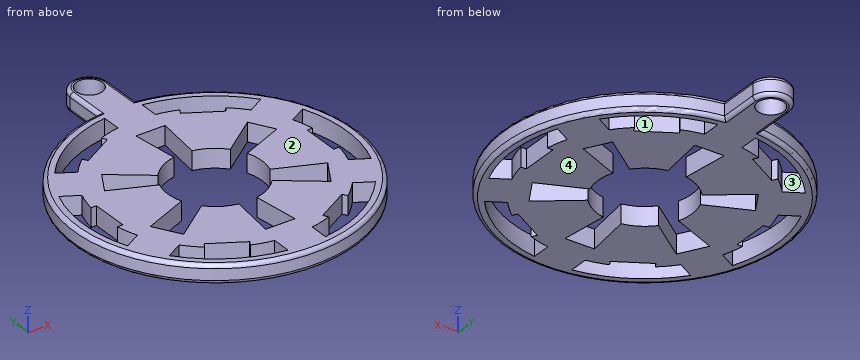
```python
from build123d import *

# Parameters (mm, degrees)
F1_DEPTH = 5
F0_R     = 3.5
F2_DEPTH = 5
F3_R     = 1


with BuildPart() as f1:
    # F0 (on Top) → F1 (new body)
    with BuildSketch(Plane.XY):
        with BuildLine():
            ThreePointArc((-4.988375268, 37.1667339456), (-24.6899364868, -28.2251135742), (37.5, 0))
            ThreePointArc((37.5, 0), (28.2251135742, 24.6899364868), (4.988375268, 37.1667339456))
            ThreePointArc((4.988375268, 37.1667339456), (0, 37.5), (-4.988375268, 37.1667339456))
        make_face()
        with BuildLine():
            Line((-5, -29.5803989155), (-5, -30))
            Line((-5, -30), (-5, -34.6410161514))
            ThreePointArc((-5, -34.6410161514), (-17.5, -30.3108891325), (-27.5, -21.6506350946))
            Line((-27.5, -21.6506350946), (-23.1173769149, -19.1203264767))
            ThreePointArc((-23.1173769149, -19.1203264767), (-21.2132034356, -21.2132034356), (-19.1203264767, -23.1173769149))
            Line((-19.1203264767, -23.1173769149), (-18.3888154764, -21.8503626961))
            Line((-18.3888154764, -21.8503626961), (-9.7285614385, -26.8503626961))
            Line((-9.7285614385, -26.8503626961), (-10.4600724388, -28.1173769149))
            ThreePointArc((-10.4600724388, -28.1173769149), (-7.7645713531, -28.9777747887), (-5, -29.5803989155))
        make_face(mode=Mode.SUBTRACT)
        with BuildLine():
            ThreePointArc((-32.5, -12.9903810568), (-35, 0), (-32.5, 12.9903810568))
            Line((-32.5, 12.9903810568), (-28.1173769149, 10.4600724388))
            ThreePointArc((-28.1173769149, 10.4600724388), (-28.9777747887, 7.7645713531), (-29.5803989155, 5))
            Line((-29.5803989155, 5), (-28.1173769149, 5))
            Line((-28.1173769149, 5), (-28.1173769149, -5))
            Line((-28.1173769149, -5), (-29.5803989155, -5))
            ThreePointArc((-29.5803989155, -5), (-28.9777747887, -7.7645713531), (-28.1173769149, -10.4600724388))
            Line((-28.1173769149, -10.4600724388), (-32.5, -12.9903810568))
        make_face(mode=Mode.SUBTRACT)
        with BuildLine():
            Line((5, -30), (5, -29.5803989155))
            ThreePointArc((5, -29.5803989155), (7.7645713531, -28.9777747887), (10.4600724388, -28.1173769149))
            Line((10.4600724388, -28.1173769149), (9.7285614385, -26.8503626961))
            Line((9.7285614385, -26.8503626961), (18.3888154764, -21.8503626961))
            Line((18.3888154764, -21.8503626961), (19.1203264767, -23.1173769149))
            ThreePointArc((19.1203264767, -23.1173769149), (21.2132034356, -21.2132034356), (23.1173769149, -19.1203264767))
            Line((23.1173769149, -19.1203264767), (27.5, -21.6506350946))
            ThreePointArc((27.5, -21.6506350946), (17.5, -30.3108891325), (5, -34.6410161514))
            Line((5, -34.6410161514), (5, -30))
        make_face(mode=Mode.SUBTRACT)
        with BuildLine():
            ThreePointArc((-9.6656079434, 7.926286841), (-6.3749366407, 10.7522175772), (-2.3166453596, 12.2834504223))
            Line((-2.3166453596, 12.2834504223), (-3.8166453596, 24.5))
            Line((-3.8166453596, 24.5), (4, 24.5))
            Line((4, 24.5), (2.5, 12.2474487139))
            ThreePointArc((2.5, 12.2474487139), (6.4551230926, 10.7042695154), (9.6656079434, 7.926286841))
            Line((9.6656079434, 7.926286841), (19.4529138373, 15.3065648785))
            Line((19.4529138373, 15.3065648785), (22.9823309481, 9.1934351215))
            Line((22.9823309481, 9.1934351215), (11.6971697336, 4.4075186015))
            ThreePointArc((11.6971697336, 4.4075186015), (12.4985113757, 0.1929077306), (11.827620909, -4.0444262427))
            Line((11.827620909, -4.0444262427), (23.6581671568, -9.040247023))
            Line((23.6581671568, -9.040247023), (19.6581671568, -15.9684502533))
            Line((19.6581671568, -15.9684502533), (9.4163863244, -8.2208070522))
            ThreePointArc((9.4163863244, -8.2208070522), (6.2891594451, -10.8026141963), (2.5, -12.2474487139))
            Line((2.5, -12.2474487139), (4, -24.5))
            Line((4, -24.5), (-3.8166453596, -24.5))
            Line((-3.8166453596, -24.5), (-2.3166453596, -12.2834504223))
            ThreePointArc((-2.3166453596, -12.2834504223), (-6.2082425785, -10.849319061), (-9.4163863244, -8.2208070522))
            Line((-9.4163863244, -8.2208070522), (-19.6581671568, -15.9684502533))
            Line((-19.6581671568, -15.9684502533), (-23.6581671568, -9.040247023))
            Line((-23.6581671568, -9.040247023), (-11.827620909, -4.0444262427))
            ThreePointArc((-11.827620909, -4.0444262427), (-12.4985113757, 0.1929077306), (-11.6971697336, 4.4075186015))
            Line((-11.6971697336, 4.4075186015), (-22.9823309481, 9.1934351215))
            Line((-22.9823309481, 9.1934351215), (-19.4529138373, 15.3065648785))
            Line((-19.4529138373, 15.3065648785), (-9.6656079434, 7.926286841))
        make_face(mode=Mode.SUBTRACT)
        with BuildLine():
            Line((28.1173769149, 10.4600724388), (32.5, 12.9903810568))
            ThreePointArc((32.5, 12.9903810568), (35, 0), (32.5, -12.9903810568))
            Line((32.5, -12.9903810568), (28.1173769149, -10.4600724388))
            ThreePointArc((28.1173769149, -10.4600724388), (28.9777747887, -7.7645713531), (29.5803989155, -5))
            Line((29.5803989155, -5), (28.1173769149, -5))
            Line((28.1173769149, -5), (28.1173769149, 5))
            Line((28.1173769149, 5), (29.5803989155, 5))
            ThreePointArc((29.5803989155, 5), (28.9777747887, 7.7645713531), (28.1173769149, 10.4600724388))
        make_face(mode=Mode.SUBTRACT)
        with BuildLine():
            Line((-5, 30), (-5, 29.5803989155))
            ThreePointArc((-5, 29.5803989155), (-7.7645713531, 28.9777747887), (-10.4600724388, 28.1173769149))
            Line((-10.4600724388, 28.1173769149), (-9.7285614385, 26.8503626961))
            Line((-9.7285614385, 26.8503626961), (-18.3888154764, 21.8503626961))
            Line((-18.3888154764, 21.8503626961), (-19.1203264767, 23.1173769149))
            ThreePointArc((-19.1203264767, 23.1173769149), (-21.2132034356, 21.2132034356), (-23.1173769149, 19.1203264767))
            Line((-23.1173769149, 19.1203264767), (-27.5, 21.6506350946))
            ThreePointArc((-27.5, 21.6506350946), (-17.5, 30.3108891325), (-5, 34.6410161514))
            Line((-5, 34.6410161514), (-5, 30))
        make_face(mode=Mode.SUBTRACT)
        with BuildLine():
            Line((5, 29.5803989155), (5, 30))
            Line((5, 30), (5, 34.6410161514))
            ThreePointArc((5, 34.6410161514), (17.5, 30.3108891325), (27.5, 21.6506350946))
            Line((27.5, 21.6506350946), (23.1173769149, 19.1203264767))
            ThreePointArc((23.1173769149, 19.1203264767), (21.2132034356, 21.2132034356), (19.1203264767, 23.1173769149))
            Line((19.1203264767, 23.1173769149), (18.3888154764, 21.8503626961))
            Line((18.3888154764, 21.8503626961), (9.7285614385, 26.8503626961))
            Line((9.7285614385, 26.8503626961), (10.4600724388, 28.1173769149))
            ThreePointArc((10.4600724388, 28.1173769149), (7.7645713531, 28.9777747887), (5, 29.5803989155))
        make_face(mode=Mode.SUBTRACT)
    extrude(amount=F1_DEPTH)

    # F0 (on Top) → F2 (join)
    with BuildSketch(Plane.XY):
        with BuildLine():
            ThreePointArc((-4.988375268, 37.1667339456), (0, 37.5), (4.988375268, 37.1667339456))
            Line((4.988375268, 37.1667339456), (4.988375268, 47.2334879431))
            ThreePointArc((4.988375268, 47.2334879431), (0, 42.5045103852), (-4.988375268, 47.2334879431))
            Line((-4.988375268, 47.2334879431), (-4.988375268, 37.1667339456))
        make_face()
        with BuildLine():
            ThreePointArc((-4.988375268, 47.2334879431), (0, 42.5045103852), (4.988375268, 47.2334879431))
            Line((4.988375268, 47.2334879431), (4.988375268, 47.7665120569))
            ThreePointArc((4.988375268, 47.7665120569), (0, 52.4954896148), (-4.988375268, 47.7665120569))
            Line((-4.988375268, 47.7665120569), (-4.988375268, 47.2334879431))
        make_face()
        with Locations((0, 47.5)):
            Circle(F0_R, mode=Mode.SUBTRACT)
    extrude(amount=F2_DEPTH)

    # F3
    f3_edges = [f1.edges().sort_by_distance(p)[0] for p in [
        (4.988375, 42.466623, 0),
        (-4.988375, 42.466623, 0),
        (4.988375, 42.466623, 5),
        (-4.988375, 42.466623, 5),
        (0, 52.49549, 5),
        (0, 52.49549, 0),
        (-24.689936, -28.225114, 0),
        (-24.689936, -28.225114, 5),
    ]]
    fillet(f3_edges, radius=F3_R)


solid = f1.part
```
Can you work these out from the model? Positions are in its coordinate system, mm. Face numbers are marked on the shaded views. A direction names the side the tool comes from. Give positions to 0.01 mm unless a question says otherwise; leave off trailing zeros. One line per item, written item: value.
1) We'd pull the mould along X, two halves only. Please class the marked faces 1 and 2: released by +X, released by -X, zero draft, split by the parting line, or undercut.
Answer sheet:
face 1: undercut
face 2: zero draft
2) On a 3-axis mill with a long thin cutter (end or side, diameter ignored), from which of +Z, -Z, +X, -X, +Y, -Y can I reach the whole of each face in a straight line? I mean the marked faces 3 and 4. Say none if no direction works.
Answer sheet:
face 3: +Z, -Z
face 4: -Z, +X, -X, +Y, -Y
3) For P1, Ø0.7, axis at x = 28.5, z = 3.5, coming from the +Y side; P2, Ø0.7, axis at x = -28.5, z = 1.5, coming from the -Y side; P3, Ø2.5, axis at y = 31, z = 2.5, coming from the -X side, each with a flat end and sliding along its axis, tell me the tip position at first contact or that it passes through.
Answer sheet:
P1: stops at y = 24.78
P2: stops at y = -24.78
P3: stops at x = -22.83
4) Please list where these lines run through material, in increasing order: line 1 along X through (y, z) = (7, 2.75); line 2 along X through (y, z) = (-15.5, 3.25); line 3 along X through (y, z) = (-31, 3.55).
Answer sheet:
line 1: x = -36.84 to -34.29, -29.17 to -17.81, 17.81 to 29.17, 34.29 to 36.84
line 2: x = -34.15 to -19.93, -19.04 to -2.71, 2.9 to 19.04, 19.93 to 34.15
line 3: x = -21.1 to -16.25, -5 to 5, 16.25 to 21.1
5) I want a section at A-A, the plane x = 0. Count the separate pieces of the cut face and the enclosed holes in it, plus the area to 3 significant figures.
Answer sheet:
separate pieces: 3
enclosed holes: 0
area: 169 mm^2
